```python
from build123d import *

# Parameters (mm, degrees)
SKETCH1_W                    = 58.25
SKETCH1_H                    = 100
BASE_FLANGE1_DEPTH           = 2.5
EDGE_FLANGE1_STRIP_W         = 11.4732
EDGE_FLANGE1_STRIP_H         = 2.5
EDGE_FLANGE1_STRIP_CUT_DEPTH = 100
EDGE_FLANGE1_DEPTH           = 100
CUT_EXTRUDE1_START           = -30
CUT_EXTRUDE1_OUTLINE_W       = 2.5
CUT_EXTRUDE1_OUTLINE_H       = 39.536796564
CUT_EXTRUDE1_OUTLINE_W_2     = 39.536796564
CUT_EXTRUDE1_OUTLINE_H_2     = 2.5
CUT_EXTRUDE1_DEPTH           = 30
CUT_EXTRUDE2_REACH           = 98.365
SKETCH21_R                   = 1.875
CIRPATTERN1_COUNT            = 2
CIRPATTERN1_ANGLE            = 90
CUT_EXTRUDE3_REACH           = 98.365
CIRPATTERN2_COUNT            = 2
CIRPATTERN2_ANGLE            = 90
CHAMFER1_SIZE                = 15


# Read off the part's stored shape, not the designer's step: Cut-Extrude1
# Sheet-metal steps are written as plain solids
with BuildPart() as part:
    # Sketch1 → Base-Flange1 (new body)
    with BuildSketch(Plane(origin=(0, 0, 0), x_dir=(1, 0, 0), z_dir=(0, 1, 0))):
        with Locations((29.125, 0)):
            Rectangle(SKETCH1_W, SKETCH1_H)
    extrude(amount=BASE_FLANGE1_DEPTH)

    # Edge-Flange1 strip (across the edge) → Edge-Flange1 strip cut (cut)
    with BuildSketch(Plane(origin=(0, 2.5, -50), x_dir=(1, 0, 0), z_dir=(0, 0, 1))):
        with Locations((-2.5, -1.25)):
            Rectangle(EDGE_FLANGE1_STRIP_W, EDGE_FLANGE1_STRIP_H)
    extrude(amount=EDGE_FLANGE1_STRIP_CUT_DEPTH, mode=Mode.SUBTRACT)

    # Edge-Flange1 section (across the edge) → Edge-Flange1 (add)
    with BuildSketch(Plane(origin=(0, 2.5, -50), x_dir=(1, 0, 0), z_dir=(0, 0, 1))):
        with BuildLine():
            Line((0, 0.7366), (0, 55.75))
            Line((0, 55.75), (2.5, 55.75))
            Line((2.5, 55.75), (2.5, 0.7366))
            ThreePointArc((2.5, 0.7366), (2.715745145, 0.215745145), (3.2366, 0))
            Line((3.2366, 0), (3.2366, -2.5))
            ThreePointArc((3.2366, -2.5), (0.947978192, -1.552021808), (0, 0.7366))
        make_face()
    extrude(amount=EDGE_FLANGE1_DEPTH)

    # Cut-Extrude1 outline → Cut-Extrude1 (cut)
    with BuildSketch(Plane.XY.offset(50).offset(CUT_EXTRUDE1_START)):
        with Locations((1.25, 38.481601718)):
            Rectangle(CUT_EXTRUDE1_OUTLINE_W, CUT_EXTRUDE1_OUTLINE_H)
        with Locations((38.481601718, 1.25)):
            Rectangle(CUT_EXTRUDE1_OUTLINE_W_2, CUT_EXTRUDE1_OUTLINE_H_2)
    cut_extrude1 = extrude(amount=CUT_EXTRUDE1_DEPTH, mode=Mode.SUBTRACT)

    # Sketch21 → Cut-Extrude2 (cut, up to next)
    with BuildSketch(Plane.XZ, mode=Mode.PRIVATE) as cut_extrude2_sk1:
        with Locations(Location((51.75, 12, 0), (0, 0, 270))):
            Circle(SKETCH21_R)
    cut_extrude2_tool1 = extrude(cut_extrude2_sk1.sketch, amount=-CUT_EXTRUDE2_REACH, mode=Mode.PRIVATE) & part.part
    # Sketch21 → Cut-Extrude2 (cut, up to next)
    with BuildSketch(Plane.XZ, mode=Mode.PRIVATE) as cut_extrude2_sk2:
        with Locations(Location((39.75, 12, 0), (0, 0, 270))):
            Circle(SKETCH21_R)
    cut_extrude2_tool2 = extrude(cut_extrude2_sk2.sketch, amount=-CUT_EXTRUDE2_REACH, mode=Mode.PRIVATE) & part.part
    cut_extrude2_1 = cut_extrude2_tool1.solids().sort_by_distance((51.75, 0, 12))[0]
    add(cut_extrude2_1, mode=Mode.SUBTRACT)
    cut_extrude2_2 = cut_extrude2_tool2.solids().sort_by_distance((39.75, 0, 12))[0]
    add(cut_extrude2_2, mode=Mode.SUBTRACT)
    cut_extrude2 = cut_extrude2_1 + cut_extrude2_2  # Cut-Extrude2 as one shape, for the pattern or mirror that repeats it

    # CirPattern1: Cut-Extrude2; each copy of Cut-Extrude2 runs up to whatever stops it at its own place
    cirpattern1_before = part.part  # the part as the pattern finds it: every copy runs up to it
    cirpattern1_cut_extrude2_long1 = extrude(cut_extrude2_sk1.sketch, amount=-CUT_EXTRUDE2_REACH, mode=Mode.PRIVATE)
    cirpattern1_cut_extrude2_long2 = extrude(cut_extrude2_sk2.sketch, amount=-CUT_EXTRUDE2_REACH, mode=Mode.PRIVATE)
    cirpattern1_cut_extrude2_tool1_1 = cirpattern1_cut_extrude2_long1.rotate(Axis((3.2366, 3.2366, 0), (0, 0, 1)), 1 * CIRPATTERN1_ANGLE / (CIRPATTERN1_COUNT - 1)) & cirpattern1_before
    add(cirpattern1_cut_extrude2_tool1_1.solids().sort_by_distance((6.4732, 51.75, 12))[0], mode=Mode.SUBTRACT)
    cirpattern1_cut_extrude2_tool2_1 = cirpattern1_cut_extrude2_long2.rotate(Axis((3.2366, 3.2366, 0), (0, 0, 1)), 1 * CIRPATTERN1_ANGLE / (CIRPATTERN1_COUNT - 1)) & cirpattern1_before
    add(cirpattern1_cut_extrude2_tool2_1.solids().sort_by_distance((6.4732, 39.75, 12))[0], mode=Mode.SUBTRACT)

    # Mirror1: Cut-Extrude1 across plane
    add(cut_extrude1.mirror(Plane.XY), mode=Mode.SUBTRACT)

    # Sketch22 → Cut-Extrude3 (cut, up to next)
    with BuildSketch(Plane.ZY, mode=Mode.PRIVATE) as cut_extrude3_sk1:
        Polygon((-20, 18.713203436), (-20, 58.25), (5, 58.25), align=None)
    cut_extrude3_tool1 = extrude(cut_extrude3_sk1.sketch, amount=-CUT_EXTRUDE3_REACH, mode=Mode.PRIVATE) & part.part
    cut_extrude3 = cut_extrude3_tool1.solids().sort_by_distance((0, 45.071068, -11.666667))[0]
    add(cut_extrude3, mode=Mode.SUBTRACT)

    # CirPattern2: Cut-Extrude3; each copy of Cut-Extrude3 runs up to whatever stops it at its own place
    cirpattern2_before = part.part  # the part as the pattern finds it: every copy runs up to it
    cirpattern2_cut_extrude3_long = extrude(cut_extrude3_sk1.sketch, amount=-CUT_EXTRUDE3_REACH, mode=Mode.PRIVATE)
    cirpattern2_cut_extrude3_tool1 = cirpattern2_cut_extrude3_long.rotate(Axis((3.2366, 3.2366, 0), (0, 0, -1)), 1 * CIRPATTERN2_ANGLE / (CIRPATTERN2_COUNT - 1)) & cirpattern2_before
    add(cirpattern2_cut_extrude3_tool1.solids().sort_by_distance((45.071068, 6.4732, -11.666667))[0], mode=Mode.SUBTRACT)

    # Chamfer1
    chamfer1_edges = [part.edges().sort_by_distance(p)[0] for p in [
        (1.25, 18.713203436, -50),
        (18.713203436, 1.25, -50),
        (1.25, 18.713203436, 50),
        (18.713203436, 1.25, 50),
    ]]
    chamfer(chamfer1_edges, length=CHAMFER1_SIZE)


solid = part.part
```
CAD build for the part. Positions are in the model's coordinates, mm. A direction names the side the tool comes from. Round coordinates to 2 decimals unless told otherwise and drop trailing zeros. Order: outer loops, then holes, each group sorted by start corner. A loop starts at its lowest first (then second) coordinate and runs counter-clockwise, first axis right, second up.
Item 1: Pin check, flat tips, straight feed: pin 1 (0.8 mm diameter, centred on y = 1.5, z = -25, fed in from +X); pin 2 (5 mm diameter, centred on x = 51.75, z = 12, fed in from +Y); pin 3 (4.5 mm diameter, centred on y = 39.75, z = 12, fed in from +X). Stop position of each tip, or through.
Item 2: Probe line 1 along Y through (x, z) = (0.7, 12) (3 decimals); line 2 along Y through (x, z) = (1, 12) (3 decimals); line 3 along X through (y, z) = (1.3, 12) (3 decimals). List the from-to ranges inside material, lowest first.
Item 3: Saw through at A-A on z = 12. Write the cut outline in (x, y) (3 decimals), then the cut area to 3 significant figures.
Item 4: Mould opens along Z. For faces 4 (the face through (1.27, 53.61, 12.24)), 5 (the face through (38.8, 1.3, -7.3)), 6 (the face through (18.713, 1, 27)), 7 (the face through (1.27, 41.61, 12.24)) say: pulls with the +Z half, pulls with the -Z half, needs draft (parallel to the pull), parting line crosses it, or undercut.
Item 5: Tool access for faces 1 (the face through (2.5, 19, -1)), 2 (the face through (18.713, 1, -27)), 3 (the face through (1, 18.713, -27)): list every direction of +Z, -Z, +X, -X, +Y, -Y with a clear straight run to the whole face (end or side of a thin tool).
Item 6: Saw through at B-B on y = 51.75. Write the cut outline in (x, z) (3 decimals).
Item 7: Saw through at D-D on x = 39.75. Write the cut outline in (y, z) (3 decimals), then the cut area to 3 significant figures.
Item 8: Saw through at C-C on z = 23. Write the cut outline in (x, y), then the cut area to 3 significant figures.
Reported:
1. pin 1: stops at x = 18.71
1. pin 2: stops at y = 2.5
1. pin 3: stops at x = 2.5
2. line 1: y = 1.226 to 37.875, 41.625 to 49.875, 53.625 to 58.25
2. line 2: y = 0.897 to 37.875, 41.625 to 49.875, 53.625 to 58.25
2. line 3: x = 0.643 to 37.875, 41.625 to 49.875, 53.625 to 58.25
3. outline: (0, 3.237) arc R3.237 ccw to (3.237, 0) - (37.875, 0) - (37.875, 2.5) - (3.237, 2.5) arc R0.737 cw to (2.5, 3.237) - (2.5, 37.875) - (0, 37.875) - close; (0, 41.625) - (2.5, 41.625) - (2.5, 49.875) - (0, 49.875) - close; (0, 53.625) - (2.5, 53.625) - (2.5, 58.25) - (0, 58.25) - close; (41.625, 0) - (49.875, 0) - (49.875, 2.5) - (41.625, 2.5) - close; (53.625, 0) - (58.25, 0) - (58.25, 2.5) - (53.625, 2.5) - close
3. area: 245 mm2
4. face 4: undercut
4. face 5: pulls with the -Z half
4. face 6: needs draft
4. face 7: undercut
5. face 1: +Z, -Z, +X, +Y
5. face 2: -Z, +X, +Y, -Y
5. face 3: -Z, +X, -X, +Y
6. outline: (0, 0.89) - (2.5, 0.89) - (2.5, 10.125) - (0, 10.125) - close; (0, 13.875) - (2.5, 13.875) - (2.5, 20) - (0, 20) - close
7. outline: (0, -6.698) - (2.5, -6.698) - (2.5, 10.125) - (0, 10.125) - close; (0, 13.875) - (2.5, 13.875) - (2.5, 20) - (0, 20) - close
7. area: 57.4 mm2
8. outline: (0, 3.24) arc R3.24 ccw to (3.24, 0) - (18.71, 0) - (18.71, 2.5) - (3.24, 2.5) arc R0.74 cw to (2.5, 3.24) - (2.5, 18.71) - (0, 18.71) - close
8. area: 85.2 mm2
